from build123d import *

# Parameters (mm, degrees)
F0_R     = 2.6543
F0_W     = 67.4656428301
F0_H     = 45.0660958886
F0_R_2   = 2.6574668283
F1_DEPTH = 5
F0_R_3   = 24.6634
F0_R_4   = 24.6579201523
F2_DEPTH = 4
F3_DEPTH = 10
F0_R_5   = 5.2850261196
F4_DEPTH = 3


# Not quite as in the source:
# - ends of sketch curves that miss each other by under 0.0002 mm in the source are joined


with BuildPart() as f1:
    # F0 (on Top) → F1 (new body)
    with BuildSketch(Plane.XY):
        with BuildLine():
            ThreePointArc((127, 43.18), (117.5777235877, 50.8), (127, 58.42))
            ThreePointArc((127, 58.42), (157.5328708116, 132.1328708116), (83.82, 101.6))
            ThreePointArc((83.82, 101.6), (63.4999991392, 81.2799974683), (43.18, 101.6))
            ThreePointArc((43.18, 101.6), (-30.5328708116, 132.1328708116), (0, 58.42))
            ThreePointArc((0, 58.42), (7.62, 50.8), (0, 43.18))
            ThreePointArc((0, 43.18), (-30.5328708116, -30.5328708116), (43.18, 0))
            ThreePointArc((43.18, 0), (63.5, 21.5136188611), (83.82, 0))
            ThreePointArc((83.82, 0), (157.5328708116, -30.5328708116), (127, 43.18))
        make_face()
        with BuildLine():
            ThreePointArc((131.5376346572, 63.7711767072), (129.2728652121, 63.5678546), (127, 63.5))
            ThreePointArc((127, 63.5), (125.778197507, 63.5195956079), (124.55765181, 63.5783622746))
            ThreePointArc((124.55765181, 63.5783622746), (112.565928289, 50.8), (124.55765181, 38.0216377254))
            ThreePointArc((124.55765181, 38.0216377254), (125.778197507, 38.0804043921), (127, 38.1))
            ThreePointArc((127, 38.1), (129.277372025, 38.0318757973), (131.5466, 37.8277468063))
            ThreePointArc((131.5466, 37.8277468063), (165.1, 0), (131.5466, -37.8277468063))
            ThreePointArc((131.5466, -37.8277468063), (129.277372025, -38.0318757973), (127, -38.1))
            ThreePointArc((127, -38.1), (100.0592316368, -26.9407683632), (88.9, 0))
            ThreePointArc((88.9, 0), (88.9063611266, 0.6961877498), (88.9254423823, 1.3921430304))
            ThreePointArc((88.9254423823, 1.3921430304), (63.5, 26.5870041852), (38.0745576177, 1.3921430304))
            ThreePointArc((38.0745576177, 1.3921430304), (38.0936388734, 0.6961877498), (38.1, 0))
            ThreePointArc((38.1, 0), (28.5029424797, -25.2822520753), (4.5466, -37.8277468063))
            ThreePointArc((4.5466, -37.8277468063), (2.277372025, -38.0318757973), (0, -38.1))
            ThreePointArc((0, -38.1), (-38.1, 0), (0, 38.1))
            ThreePointArc((0, 38.1), (12.7, 50.8), (0, 63.5))
            ThreePointArc((0, 63.5), (-38.1, 101.6), (0, 139.7))
            ThreePointArc((0, 139.7), (2.277372025, 139.6318757973), (4.5466, 139.4277468063))
            ThreePointArc((4.5466, 139.4277468063), (28.5029424797, 126.8822520753), (38.1, 101.6))
            ThreePointArc((38.1, 101.6), (63.5, 76.1999974683), (88.9, 101.6))
            ThreePointArc((88.9, 101.6), (99.7497914455, 128.2277324182), (126.1197445529, 139.6898300121))
            ThreePointArc((126.1197445529, 139.6898300121), (128.3955342395, 139.6744334716), (130.6663445529, 139.5231844341))
            ThreePointArc((130.6663445529, 139.5231844341), (165.097480066, 102.0381924437), (131.5376346572, 63.7711767072))
        make_face(mode=Mode.SUBTRACT)
        with BuildLine():
            ThreePointArc((0, 63.5), (2.277372025, 63.5681242027), (4.5466, 63.7722531937))
            Line((4.5466, 63.7722531937), (4.5466, 73.7106698774))
            ThreePointArc((4.5466, 73.7106698774), (2.2807411415, 73.4346928635), (0, 73.3425))
            Line((0, 73.3425), (0, 63.5))
        make_face()
        with BuildLine():
            Line((4.5466, 129.4893301226), (4.5466, 139.4277468063))
            ThreePointArc((4.5466, 139.4277468063), (2.277372025, 139.6318757973), (0, 139.7))
            Line((0, 139.7), (0, 129.8575))
            ThreePointArc((0, 129.8575), (2.2807411415, 129.7653071365), (4.5466, 129.4893301226))
        make_face()
        with BuildLine():
            Line((4.5466, 27.8240290125), (4.5466, 37.8277468063))
            ThreePointArc((4.5466, 37.8277468063), (2.277372025, 38.0318757973), (0, 38.1))
            Line((0, 38.1), (0, 28.1930516626))
            ThreePointArc((0, 28.1930516626), (2.2807755959, 28.1006445607), (4.5466, 27.8240290125))
        make_face()
        with BuildLine():
            ThreePointArc((0, -38.1), (2.277372025, -38.0318757973), (4.5466, -37.8277468063))
            Line((4.5466, -37.8277468063), (4.5466, -27.8240290125))
            ThreePointArc((4.5466, -27.8240290125), (2.2807755959, -28.1006445607), (0, -28.1930516626))
            Line((0, -28.1930516626), (0, -38.1))
        make_face()
        with BuildLine():
            ThreePointArc((124.55765181, 38.0216377254), (112.565928289, 50.8), (124.55765181, 63.5783622746))
            ThreePointArc((124.55765181, 63.5783622746), (99.2091429959, 75.5370326521), (88.9, 101.6))
            ThreePointArc((88.9, 101.6), (63.5, 76.1999974683), (38.1, 101.6))
            ThreePointArc((38.1, 101.6), (28.5029424797, 76.3177479247), (4.5466, 63.7722531937))
            ThreePointArc((4.5466, 63.7722531937), (2.277372025, 63.5681242027), (0, 63.5))
            ThreePointArc((0, 63.5), (12.7, 50.8), (0, 38.1))
            ThreePointArc((0, 38.1), (2.277372025, 38.0318757973), (4.5466, 37.8277468063))
            ThreePointArc((4.5466, 37.8277468063), (28.0362100648, 25.7988551142), (38.0745576177, 1.3921430304))
            ThreePointArc((38.0745576177, 1.3921430304), (63.5, 26.5870041852), (88.9254423823, 1.3921430304))
            ThreePointArc((88.9254423823, 1.3921430304), (99.6900222545, 26.566428355), (124.55765181, 38.0216377254))
        make_face()
        with Locations((38.6349633336, 18.2641260326)):
            Circle(F0_R, mode=Mode.SUBTRACT)
        with Locations((13.3296269923, 40.3755865991)):
            Circle(F0_R, mode=Mode.SUBTRACT)
        with Locations((88.0172178149, 18.018445)):
            Circle(F0_R, mode=Mode.SUBTRACT)
        with Locations((112.3398169875, 40.3755865991)):
            Circle(F0_R, mode=Mode.SUBTRACT)
        with Locations((13.0839459598, 61.2586289644)):
            Circle(F0_R, mode=Mode.SUBTRACT)
        with Locations((38.8806462288, 84.1071307659)):
            Circle(F0_R, mode=Mode.SUBTRACT)
        with Locations((63.501621415, 52.8839789331)):
            Rectangle(F0_W, F0_H, mode=Mode.SUBTRACT)
        with Locations((112.8311827779, 61.2586289644)):
            Circle(F0_R, mode=Mode.SUBTRACT)
        with Locations((87.9784226418, 84.1848701239)):
            Circle(F0_R_2, mode=Mode.SUBTRACT)
        with BuildLine():
            Line((130.6663445529, 129.6087763106), (130.6663445529, 139.5231844341))
            ThreePointArc((130.6663445529, 139.5231844341), (128.3955342395, 139.6744334716), (126.1197445529, 139.6898300121))
            Line((126.1197445529, 139.6898300121), (126.1197445529, 129.8340004808))
            ThreePointArc((126.1197445529, 129.8340004808), (128.3975888552, 129.8131242189), (130.6663445529, 129.6087763106))
        make_face()
        with BuildLine():
            Line((127, 73.3522809275), (127, 63.5))
            ThreePointArc((127, 63.5), (129.2728652121, 63.5678546), (131.5376346572, 63.7711767072))
            Line((131.5376346572, 63.7711767072), (131.5376346572, 73.7191193733))
            ThreePointArc((131.5376346572, 73.7191193733), (129.2762193835, 73.4441398974), (127, 73.3522809275))
        make_face()
        with BuildLine():
            ThreePointArc((131.5466, 37.8277468063), (129.277372025, 38.0318757973), (127, 38.1))
            Line((127, 38.1), (127, 28.3257955932))
            ThreePointArc((127, 28.3257955932), (129.2807048906, 28.2338286668), (131.5466, 27.958525076))
            Line((131.5466, 27.958525076), (131.5466, 37.8277468063))
        make_face()
        with BuildLine():
            ThreePointArc((127, -38.1), (129.277372025, -38.0318757973), (131.5466, -37.8277468063))
            Line((131.5466, -37.8277468063), (131.5466, -27.958525076))
            ThreePointArc((131.5466, -27.958525076), (129.2807048906, -28.2338286668), (127, -28.3257955932))
            Line((127, -28.3257955932), (127, -38.1))
        make_face()
    extrude(amount=F1_DEPTH)

    # F0 (on Top) → F2 (join)
    with BuildSketch(Plane.XY):
        with BuildLine():
            ThreePointArc((28.1930516626, 0), (21.4829082149, 18.2574044344), (4.5466, 27.8240290125))
            ThreePointArc((4.5466, 27.8240290125), (2.2807755959, 28.1006445607), (0, 28.1930516626))
            ThreePointArc((0, 28.1930516626), (-28.1930516626, 0), (0, -28.1930516626))
            ThreePointArc((0, -28.1930516626), (2.2807755959, -28.1006445607), (4.5466, -27.8240290125))
            ThreePointArc((4.5466, -27.8240290125), (21.4829082149, -18.2574044344), (28.1930516626, 0))
        make_face()
        Circle(F0_R_3, mode=Mode.SUBTRACT)
        with BuildLine():
            ThreePointArc((28.2575, 101.6), (21.5286071977, 119.9031521431), (4.5466, 129.4893301226))
            ThreePointArc((4.5466, 129.4893301226), (2.2807411415, 129.7653071365), (0, 129.8575))
            ThreePointArc((0, 129.8575), (-28.2575, 101.6), (0, 73.3425))
            ThreePointArc((0, 73.3425), (2.2807411415, 73.4346928635), (4.5466, 73.7106698774))
            ThreePointArc((4.5466, 73.7106698774), (21.5286071977, 83.2968478569), (28.2575, 101.6))
        make_face()
        with Locations((0, 101.6)):
            Circle(F0_R_3, mode=Mode.SUBTRACT)
        with BuildLine():
            ThreePointArc((126.1197445529, 129.8340004808), (98.7557107836, 101.1598188294), (127, 73.3522809275))
            ThreePointArc((127, 73.3522809275), (129.2762193835, 73.4441398974), (131.5376346572, 73.7191193733))
            ThreePointArc((131.5376346572, 73.7191193733), (148.5187297703, 83.3003305528), (155.2477190725, 101.6))
            ThreePointArc((155.2477190725, 101.6), (148.2308679021, 120.2328709791), (130.6663445529, 129.6087763106))
            ThreePointArc((130.6663445529, 129.6087763106), (128.3975888552, 129.8131242189), (126.1197445529, 129.8340004808))
        make_face()
        with Locations((127, 101.6)):
            Circle(F0_R_3, mode=Mode.SUBTRACT)
        with BuildLine():
            ThreePointArc((131.5466, 27.958525076), (129.2807048906, 28.2338286668), (127, 28.3257955932))
            ThreePointArc((127, 28.3257955932), (98.6742044068, 0), (127, -28.3257955932))
            ThreePointArc((127, -28.3257955932), (129.2807048906, -28.2338286668), (131.5466, -27.958525076))
            ThreePointArc((131.5466, -27.958525076), (148.5770336032, -18.3516298151), (155.3257955932, 0))
            ThreePointArc((155.3257955932, 0), (148.5770336032, 18.3516298151), (131.5466, 27.958525076))
        make_face()
        with Locations((127, 0)):
            Circle(F0_R_4, mode=Mode.SUBTRACT)
    extrude(amount=F2_DEPTH)

    # F3 (add): faces of the model
    f3_faces = [f1.faces().sort_by_distance(p)[0] for p in [
        (2.2162320404, 128.9686719497, 4),
        (129.2118381771, 74.2405078817, 4),
        (129.2161968149, 27.4352553985, 4),
        (27.3956317421, 0, 4),
    ]]
    extrude(f3_faces, amount=F3_DEPTH)

    # F0 (on Top) → F4 (join)
    with BuildSketch(Plane.XY):
        with Locations((63.501621415, 52.8839789331)):
            Rectangle(F0_W, F0_H)
        with Locations((39.8230690813, 37.1708342285)):
            Circle(F0_R_5, mode=Mode.SUBTRACT)
        with Locations((52.241603622, 36.8332513428)):
            Circle(F0_R_5, mode=Mode.SUBTRACT)
        with Locations((39.5965345407, 47.9224171143)):
            Circle(F0_R_5, mode=Mode.SUBTRACT)
        with Locations((52.0150690813, 47.5848342285)):
            Circle(F0_R_5, mode=Mode.SUBTRACT)
        with Locations((64.6601381626, 36.495668457)):
            Circle(F0_R_5, mode=Mode.SUBTRACT)
        with Locations((77.0786727033, 36.1580855713)):
            Circle(F0_R_5, mode=Mode.SUBTRACT)
        with Locations((89.4972072439, 35.8205026855)):
            Circle(F0_R_5, mode=Mode.SUBTRACT)
        with Locations((64.433603622, 47.2472513428)):
            Circle(F0_R_5, mode=Mode.SUBTRACT)
        with Locations((76.8521381626, 46.909668457)):
            Circle(F0_R_5, mode=Mode.SUBTRACT)
        with Locations((89.2706727033, 46.5720855713)):
            Circle(F0_R_5, mode=Mode.SUBTRACT)
        with Locations((39.37, 58.674)):
            Circle(F0_R_5, mode=Mode.SUBTRACT)
        with Locations((51.7885345407, 58.3364171143)):
            Circle(F0_R_5, mode=Mode.SUBTRACT)
        with Locations((39.1434654593, 69.4255828857)):
            Circle(F0_R_5, mode=Mode.SUBTRACT)
        with Locations((51.562, 69.088)):
            Circle(F0_R_5, mode=Mode.SUBTRACT)
        with Locations((64.2070690813, 57.9988342285)):
            Circle(F0_R_5, mode=Mode.SUBTRACT)
        with Locations((76.625603622, 57.6612513428)):
            Circle(F0_R_5, mode=Mode.SUBTRACT)
        with Locations((89.0441381626, 57.323668457)):
            Circle(F0_R_5, mode=Mode.SUBTRACT)
        with Locations((76.3990690813, 68.4128342285)):
            Circle(F0_R_5, mode=Mode.SUBTRACT)
        with Locations((63.9805345407, 68.7504171143)):
            Circle(F0_R_5, mode=Mode.SUBTRACT)
        with Locations((88.817603622, 68.0752513428)):
            Circle(F0_R_5, mode=Mode.SUBTRACT)
    extrude(amount=F4_DEPTH)


solid = f1.part
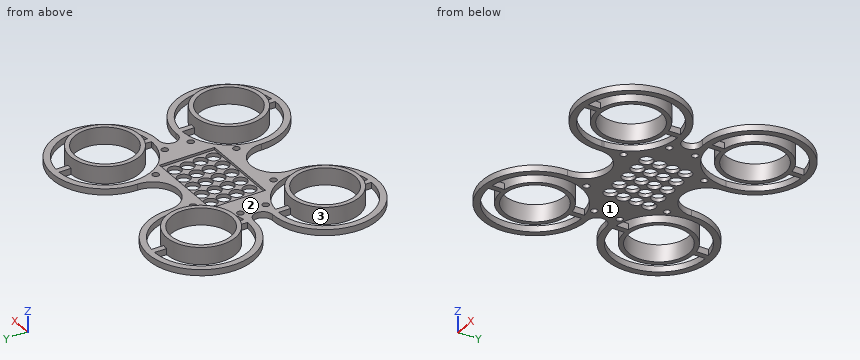
Model file for the job. Use its own axes, mm. Face numbers are marked on the shaded views. Give positions to 0.01 mm unless a question says otherwise; leave off trailing zeros. Loops run counter-clockwise (first coordinate to the right, second up) from the corner with the lowest first, then second, coordinate; pieces in that order, holes last.
1) Flat gauge pins, fed straight in: pin 1 Ø9.5 at (x, y) = (64.43, 47.25) entering from -Z; pin 2 Ø2.5 at (y, z) = (136, 3.5) entering from +X; pin 3 Ø5 at (y, z) = (81.5, 2) entering from +X; pin 4 Ø3 at (y, z) = (38.5, 4) entering from -X. Where does each tip first touch, or does it go through?
2) Saw through at B-B (x = 63.5). Write the cut outline in (y, z), plus the area to 3 significant figures.
3) Pull direction X, two halves, no side cores. Call the marked faces 1, 2 and 3: +X half, -X half, draft (parallel to the pull), parting line (faces both ways), or undercut.
4) Saw through at A-A (z = 10.25). Write the cut outline in (x, y) (1 decimal).
5) Wall check: line 1 (Y direction, x = 127, z = 11.5); line 2 (Y direction, x = 8, z = 7); line 3 (Z direction, x = 47.5, y = 30). Give the ranges that are in metal, low to high.
Answer block:
1. pin 1: passes through
1. pin 2: stops at x = 154.67
1. pin 3: stops at x = 166.43
1. pin 4: stops at x = -22.26
2. outline: (21.51, 0) - (31.34, 0) - (31.34, 3) - (30.35, 3) - (30.35, 5) - (21.51, 5) - close; (41.65, 0) - (42.05, 0) - (42.05, 3) - (41.65, 3) - close; (52.45, 0) - (52.76, 0) - (52.76, 3) - (52.45, 3) - close; (63.24, 0) - (63.49, 0) - (63.49, 3) - (63.24, 3) - close; (74.01, 0) - (81.28, 0) - (81.28, 5) - (75.42, 5) - (75.42, 3) - (74.01, 3) - close
2. area: 83.5 mm2
3. face 1: draft
3. face 2: undercut
3. face 3: undercut
4. outline: circle Ø56.5 at (0, 101.6); circle Ø56.4 at (0, 0); circle Ø56.7 at (127, 0); circle Ø56.5 at (127, 101.6); hole circle Ø49.3 at (0, 0); hole circle Ø49.3 at (0, 101.6); hole circle Ø49.3 at (127, 0); hole circle Ø49.3 at (127, 101.6)
5. line 1: y = -28.33 to -24.66, 24.66 to 28.33, 73.35 to 76.94, 126.26 to 129.85
5. line 2: y = -27.03 to -23.33, 23.33 to 27.03, 74.5 to 78.27, 124.93 to 128.7
5. line 3: z = 0 to 5
